Verification items for the finished model (mm, model axes). A direction names the side the tool comes from. Coordinates: 2 decimals unless noted, no trailing zeros. Order: outer loops, then holes, each group sorted by start corner. A loop starts at its lowest first (then second) coordinate and runs counter-clockwise, first axis right, second up. Notation, with made-up numbers: M -17.5,-29.75 L -8.5,-29.75 A32 ccw -8.5,8.25 Z; hole C 86.25,-29.75 d8. An arc over 180 degrees is marked long. Write item = value, one per line.
```python
from build123d import *

# Parameters (mm, degrees)
EXTRUDE_THIN1_DEPTH        = 42.4
CUT_EXTRUDE1_REACH         = 48.479
SZKIC1_R                   = 1.6
WYTNIJ_WYCI_GNI_CIE1_DEPTH = 47.478597225


with BuildPart() as part:
    # Sketch1 → Extrude-Thin1 (new body)
    with BuildSketch(Plane(origin=(0, 0, 0), x_dir=(0, 0, -1), z_dir=(1, 0, 0))):
        with BuildLine():
            Line((-17.5, 6.5), (-15.5, 6.5))
            ThreePointArc((-15.5, 6.5), (-14.085786438, 5.914213562), (-13.5, 4.5))
            Line((-13.5, 4.5), (-13.5, 2))
            ThreePointArc((-13.5, 2), (-12.914213562, 0.585786438), (-11.5, 0))
            Line((-11.5, 0), (11.5, 0))
            ThreePointArc((11.5, 0), (12.914213562, 0.585786438), (13.5, 2))
            Line((13.5, 2), (13.5, 4.5))
            ThreePointArc((13.5, 4.5), (14.085786438, 5.914213562), (15.5, 6.5))
            Line((15.5, 6.5), (17.5, 6.5))
            Line((17.5, 6.5), (17.5, 7.5))
            Line((17.5, 7.5), (15.5, 7.5))
            ThreePointArc((15.5, 7.5), (13.378679656, 6.621320344), (12.5, 4.5))
            Line((12.5, 4.5), (12.5, 2))
            ThreePointArc((12.5, 2), (12.207106781, 1.292893219), (11.5, 1))
            Line((11.5, 1), (-11.5, 1))
            ThreePointArc((-11.5, 1), (-12.207106781, 1.292893219), (-12.5, 2))
            Line((-12.5, 2), (-12.5, 4.5))
            ThreePointArc((-12.5, 4.5), (-13.378679656, 6.621320344), (-15.5, 7.5))
            Line((-15.5, 7.5), (-17.5, 7.5))
            Line((-17.5, 7.5), (-17.5, 6.5))
        make_face()
    extrude(amount=EXTRUDE_THIN1_DEPTH)

    # Sketch2 → Cut-Extrude1 (cut, up to next)
    with BuildSketch(Plane.XZ, mode=Mode.PRIVATE) as cut_extrude1_sk1:
        with BuildLine():
            Line((-5.875, 3.125), (5.875, 3.125))
            ThreePointArc((5.875, 3.125), (9, 0), (5.875, -3.125))
            Line((5.875, -3.125), (-5.875, -3.125))
            ThreePointArc((-5.875, -3.125), (-9, 0), (-5.875, 3.125))
        make_face()
    cut_extrude1_tool1 = extrude(cut_extrude1_sk1.sketch, amount=-CUT_EXTRUDE1_REACH, mode=Mode.PRIVATE) & part.part
    add(cut_extrude1_tool1.solids().sort_by_distance((0, 0, 0))[0], mode=Mode.SUBTRACT)

    # Szkic1 → Wytnij-wyciągnięcie1 (cut, through all)
    with BuildSketch(Plane.XZ):
        with Locations(Location((35.396484606, 0, 0), (0, 0, 270))):
            Circle(SZKIC1_R)
        with Locations(Location((21.2, 0, 0), (0, 0, 270))):
            Circle(SZKIC1_R)
    extrude(amount=-WYTNIJ_WYCI_GNI_CIE1_DEPTH, mode=Mode.SUBTRACT)


solid = part.part
```
Item 1: Sectioned sample at C-C, the plane x = 21.2. Enter the section's corners in (y, z).
Report:
outline = M 0,-11.5 A2 ccw 2,-13.5 L 4.5,-13.5 A2 cw 6.5,-15.5 L 6.5,-17.5 L 7.5,-17.5 L 7.5,-15.5 A3 ccw 4.5,-12.5 L 2,-12.5 A1 cw 1,-11.5 L 1,-1.6 L 0,-1.6 Z; M 0,1.6 L 1,1.6 L 1,11.5 A1 cw 2,12.5 L 4.5,12.5 A3 ccw 7.5,15.5 L 7.5,17.5 L 6.5,17.5 L 6.5,15.5 A2 cw 4.5,13.5 L 2,13.5 A2 ccw 0,11.5 Z
Item 2: Tool access check on faces 1 (the flat face through (21, 6.5, 17)), 2 (the flat face through (21, 1, -3)), 3 (the cylindrical face through (19.64, 0.49, 0.35)). Record the directions out of +Z, -Z, +X, -X, +Y, -Y that give a thin tool (end or side, any length) a straight path to the whole face; none if there is none.
Report:
face_1 = +Z, +X, -X, -Y
face_2 = +X, -X, +Y
face_3 = +Y, -Y
Item 3: Gauge pin test, flat ends, axial feed: pin 1 (0.8 mm diameter, centred on x = 11.5, y = 3, fed in from +Z); pin 2 (3 mm diameter, centred on x = 26, y = 3, fed in from -Z); pin 3 (1.6 mm diameter, centred on x = 21.5, z = -16, fed in from -Y). Record the tip position at first contact, or that the pin passes through.
Report:
pin_1 = 13.5
pin_2 = -13.5
pin_3 = 6.48
Item 4: Sectioned sample at B-B, the plane z = 0. Enter the section's corners in (x, y), then the cut area to 3 significant figures.
Report:
outline = M 9,0 L 19.6,0 L 19.6,1 L 9,1 Z; M 22.8,0 L 33.8,0 L 33.8,1 L 22.8,1 Z; M 37,0 L 42.4,0 L 42.4,1 L 37,1 Z
area = 27.0 mm^2
Item 5: Sectioned sample at A-A, the plane y = 2.75. Enter the section's corners in (x, z), then the cut area to 3 significant figures.
Report:
outline = M 0,-13.5 L 42.4,-13.5 L 42.4,-12.5 L 0,-12.5 Z; M 0,12.5 L 42.4,12.5 L 42.4,13.5 L 0,13.5 Z
area = 84.8 mm^2
Item 6: Scan lines: L1, parallel to X at y = 0.3, z = 0; L2, parallel to Z at x = 41.5, y = 4.25; L3, parallel to Z at x = 40, y = 1.25. Record each from-to range of solid material in increasing order. Write a range as from..to.
Report:
L1 = 9..19.6, 22.8..33.8, 37..42.4
L2 = -13.5..-12.5, 12.5..13.5
L3 = -13.35..-12.16, 12.16..13.35
Item 7: Sectioned sample at D-D, the plane x = 9.5. Enter the section's corners in (y, z).
Report:
outline = M 0,-11.5 A2 ccw 2,-13.5 L 4.5,-13.5 A2 cw 6.5,-15.5 L 6.5,-17.5 L 7.5,-17.5 L 7.5,-15.5 A3 ccw 4.5,-12.5 L 2,-12.5 A1 cw 1,-11.5 L 1,11.5 A1 cw 2,12.5 L 4.5,12.5 A3 ccw 7.5,15.5 L 7.5,17.5 L 6.5,17.5 L 6.5,15.5 A2 cw 4.5,13.5 L 2,13.5 A2 ccw 0,11.5 Z
Item 8: Release check for a two-part mould opening along Z. For faces 4 (the flat face through (21, 6.5, -16)), 5 (the flat face through (21, 3, -13.5)), 6 (the flat face through (2.9, 0.5, 3.125)), 7 (the cylindrical face through (20.9, 5.93, 14.1)) record: pulls with the +Z half, pulls with the -Z half, needs draft (parallel to the pull), parting line crosses it, or undercut.
Report:
face_4 = needs draft
face_5 = pulls with the -Z half
face_6 = undercut
face_7 = pulls with the +Z half
